from build123d import *

# Parameters (mm, degrees)
RESSALTO_EXTRUS_O1_DEPTH = 5
ESBO_O2_R                = 1.5
CORTE_EXTRUS_O1_DEPTH    = 5
ESBO_O3_R                = 1.5
CORTE_EXTRUS_O2_DEPTH    = 10


with BuildPart() as part:
    # Esboço1 → Ressalto-extrusão1 (new body)
    with BuildSketch(Plane(origin=(0, 0, 0), x_dir=(1, 0, 0), z_dir=(0, 1, 0))):
        with BuildLine():
            Line((57.825671094, 13.599370915), (57.079704402, 13.599370915))
            ThreePointArc((57.079704402, 13.599370915), (55.665490839, 14.185157352), (55.079704402, 15.599370915))
            Line((55.079704402, 15.599370915), (55.079704402, 115.599370915))
            ThreePointArc((55.079704402, 115.599370915), (55.665490839, 117.013584477), (57.079704402, 117.599370915))
            Line((57.079704402, 117.599370915), (57.825671094, 117.599370915))
            ThreePointArc((57.825671094, 117.599370915), (59.406809924, 118.374626043), (59.762162767, 120.099370915))
            ThreePointArc((59.762162767, 120.099370915), (56.203428759, 125.505065065), (50.079704402, 127.599370915))
            Line((50.079704402, 127.599370915), (-29.920295598, 127.599370915))
            ThreePointArc((-29.920295598, 127.599370915), (-36.044019955, 125.505065065), (-39.602753964, 120.099370915))
            ThreePointArc((-39.602753964, 120.099370915), (-39.247401121, 118.374626043), (-37.666262291, 117.599370915))
            Line((-37.666262291, 117.599370915), (-36.920295598, 117.599370915))
            ThreePointArc((-36.920295598, 117.599370915), (-35.506082036, 117.013584477), (-34.920295598, 115.599370915))
            Line((-34.920295598, 115.599370915), (-34.920295598, 15.599370915))
            ThreePointArc((-34.920295598, 15.599370915), (-35.506082036, 14.185157352), (-36.920295598, 13.599370915))
            Line((-36.920295598, 13.599370915), (-37.666262291, 13.599370915))
            ThreePointArc((-37.666262291, 13.599370915), (-39.247401121, 12.824115786), (-39.602753964, 11.099370915))
            ThreePointArc((-39.602753964, 11.099370915), (-36.044019955, 5.693676764), (-29.920295598, 3.599370915))
            Line((-29.920295598, 3.599370915), (50.079704402, 3.599370915))
            ThreePointArc((50.079704402, 3.599370915), (56.203428759, 5.693676764), (59.762162767, 11.099370915))
            ThreePointArc((59.762162767, 11.099370915), (59.406809924, 12.824115786), (57.825671094, 13.599370915))
        make_face()
    extrude(amount=RESSALTO_EXTRUS_O1_DEPTH)

    # Esboço2 → Corte-extrusão1 (cut)
    with BuildSketch(Plane(origin=(0, 5, 0), x_dir=(1, 0, 0), z_dir=(0, 1, 0))):
        with Locations(Location((10.079704402, 24.599370915, 0), (0, 0, 270))):
            Circle(ESBO_O2_R)
        with Locations(Location((10.079704402, 40.599370915, 0), (0, 0, 270))):
            Circle(ESBO_O2_R)
        with Locations(Location((10.079704402, 90.599370915, 0), (0, 0, 90))):
            Circle(ESBO_O2_R)
        with Locations(Location((10.079704402, 106.599370915, 0), (0, 0, 90))):
            Circle(ESBO_O2_R)
        with BuildLine():
            Line((13.579704402, 96.099370915), (13.579704402, 101.099370915))
            ThreePointArc((13.579704402, 101.099370915), (13.286811183, 101.806477696), (12.579704402, 102.099370915))
            Line((12.579704402, 102.099370915), (7.579704402, 102.099370915))
            ThreePointArc((7.579704402, 102.099370915), (6.872597621, 101.806477696), (6.579704402, 101.099370915))
            Line((6.579704402, 101.099370915), (6.579704402, 96.099370915))
            ThreePointArc((6.579704402, 96.099370915), (6.872597621, 95.392264133), (7.579704402, 95.099370915))
            Line((7.579704402, 95.099370915), (12.579704402, 95.099370915))
            ThreePointArc((12.579704402, 95.099370915), (13.286811183, 95.392264133), (13.579704402, 96.099370915))
        make_face()
        with BuildLine():
            Line((7.579704402, 36.099370915), (12.579704402, 36.099370915))
            ThreePointArc((12.579704402, 36.099370915), (13.286811183, 35.806477696), (13.579704402, 35.099370915))
            Line((13.579704402, 35.099370915), (13.579704402, 30.099370915))
            ThreePointArc((13.579704402, 30.099370915), (13.286811183, 29.392264133), (12.579704402, 29.099370915))
            Line((12.579704402, 29.099370915), (7.579704402, 29.099370915))
            ThreePointArc((7.579704402, 29.099370915), (6.872597621, 29.392264133), (6.579704402, 30.099370915))
            Line((6.579704402, 30.099370915), (6.579704402, 35.099370915))
            ThreePointArc((6.579704402, 35.099370915), (6.872597621, 35.806477696), (7.579704402, 36.099370915))
        make_face()
    extrude(amount=-CORTE_EXTRUS_O1_DEPTH, mode=Mode.SUBTRACT)

    # Esboço3 → Corte-extrusão2 (cut)
    with BuildSketch(Plane(origin=(0, 5, 0), x_dir=(1, 0, 0), z_dir=(0, 1, 0))):
        with Locations(Location((-27.920295598, 10.599370915, 0), (0, 0, 270))):
            Circle(ESBO_O3_R)
        with Locations(Location((48.079704402, 10.599370915, 0), (0, 0, 270))):
            Circle(ESBO_O3_R)
        with Locations(Location((-27.920295598, 120.599370915, 0), (0, 0, 270))):
            Circle(ESBO_O3_R)
        with Locations(Location((48.079704402, 120.599370915, 0), (0, 0, 270))):
            Circle(ESBO_O3_R)
    extrude(amount=-CORTE_EXTRUS_O2_DEPTH, mode=Mode.SUBTRACT)


solid = part.part
Geometry: final body of the model. Coordinates: model frame, mm. A direction names the side the tool comes from. Coordinates: 2 decimals unless noted, no trailing zeros. Order: outer loops, then holes, each group sorted by start corner. A loop starts at its lowest first (then second) coordinate and runs counter-clockwise, first axis right, second up.
(1) Material intervals for probe 1 along Z at (x, y) = (12, 4.3); probe 2 along Z at (x, y) = (-30, 1.75); probe 3 along X at (y, z) = (3.6, -112), sorted ascending.
(2) Draft query along X for faces 3 (the face through (56.13, 2.465, -5.638)), 4 (the face through (10.1, 2.5, -26.1)), 5 (the face through (-35.97, 2.46, -125.56)), 6 (the face through (6.58, 3, -33)). Return one class per face: pulls with the +X half, pulls with the -X half, needs draft (parallel to the pull), parting line crosses it, or undercut.
(3) Section query B-B (y = 1.6). State how many separate pieces and enclosed holes the cut face has, plus the area to 3 significant figures.
(4) Section query A-A (z = -49.5). Return the cut outline in (x, y).
(5) First-contact query: pin 1 (3 mm diameter, centred on x = 14, z = -101, fed in from -Y); pin 2 (3 mm diameter, centred on y = 1, z = -71.5, fed in from -X); pin 3 (0.6 mm diameter, centred on x = -37.5, y = 3, fed in from -Z). Flat tips, straight axial feed; report the tip coordinate or a pass-through.
(6) Access query for faces 1 (the face through (13.58, 3, -99)), 2 (the face through (-36.117, 2.465, -5.751)). Directions: +Z, -Z, +X, -X, +Y, -Y. A direction counts if a zero-diameter tool reaches every point of the face in a straight line with its end or side. Return the directions, or none.
Solution:
1. probe 1: z = -127.6 to -102.1, -95.1 to -36.1, -29.1 to -3.6
1. probe 2: z = -127.6 to -3.6
1. probe 3: x = -34.92 to 55.08
2. face 3: pulls with the +X half
2. face 4: undercut
2. face 5: pulls with the -X half
2. face 6: undercut
3. separate pieces: 1
3. enclosed holes: 10
3. area: 11,100 mm2
4. outline: (-34.92, 0) - (55.08, 0) - (55.08, 5) - (-34.92, 5) - close
5. pin 1: stops at y = 0
5. pin 2: stops at x = -34.92
5. pin 3: stops at z = -124.46
6. face 1: +Y, -Y
6. face 2: +Z, -X, +Y, -Y
